For this review, take the finished solid that the model builds, in its own axes (mm). Coordinates: 2 decimals unless noted, no trailing zeros. Use a Markdown table: item, result.
from build123d import *

# Parameters (mm, degrees)
SKETCH_1_R          = 13.5
EXTRUDE_1_DEPTH     = 2
SKETCH_2_R          = 6.25
SKETCH_2_R_2        = 1.5
SKETCH_2_R_3        = 4.25
CUT_EXTRUDE_2_DEPTH = 135.372484569
SKETCH_3_R          = 1.5
CUT_EXTRUDE_3_DEPTH = 135.372484569


with BuildPart() as part:
    # 草图1 → 凸台-拉伸1 (new body)
    with BuildSketch(Plane.XY):
        Circle(SKETCH_1_R)
        with BuildLine():
            ThreePointArc((5.892711217, -11.0238811), (8.326059469, 9.323450741), (-11.617581648, 4.613219771))
            add(Edge.make_bspline(
                [(-44.514894976, -15.648119029), (-23.754992487, -12.049932399), (-11.617581648, 4.613219771)],
                knots=[0, 0, 0, 1, 1, 1], degree=2))
            add(Edge.make_bspline(
                [(-44.514894976, -15.648119029), (-60.493246192, -16.620966096), (-98.719374485, 13.99401616), (-101.099323327, 34.577284328)],
                knots=[0, 0, 0, 0, 1, 1, 1, 1], degree=3))
            ThreePointArc((-101.099323327, 34.577284328), (-119.514224633, 44.92723863), (-120.988196928, 23.854565571))
            add(Edge.make_bspline(
                [(-43.715031798, -30.941916126), (-74.6558876, -29.772176263), (-107.934743734, 0.909272839), (-120.988196928, 23.854565571)],
                knots=[0, 0, 0, 0, 1, 1, 1, 1], degree=3))
            add(Edge.make_bspline(
                [(5.892711217, -11.0238811), (-16.208282922, -27.819747246), (-43.715031798, -30.941916126)],
                knots=[0, 0, 0, 1, 1, 1], degree=2))
        make_face()
    extrude(amount=EXTRUDE_1_DEPTH)

    # 草图2 → 切除-拉伸2 (cut, through all)
    with BuildSketch(Plane.XY):
        Circle(SKETCH_2_R)
        with Locations((-7.071067812, 7.071067812)):
            Circle(SKETCH_2_R_2)
        with Locations((7.071067812, 7.071067812)):
            Circle(SKETCH_2_R_2)
        with Locations((7.071067812, -7.071067812)):
            Circle(SKETCH_2_R_2)
        with Locations((-7.071067812, -7.071067812)):
            Circle(SKETCH_2_R_2)
        with Locations((-113.582262859, 33.924428557)):
            Circle(SKETCH_2_R_3)
        with Locations((-106.728711554, 35.34880018)):
            Circle(SKETCH_2_R_2)
        with Locations((-112.157891236, 27.070877253)):
            Circle(SKETCH_2_R_2)
        with Locations((-120.435814163, 32.500056934)):
            Circle(SKETCH_2_R_2)
        with Locations((-115.006634481, 40.777979862)):
            Circle(SKETCH_2_R_2)
    extrude(amount=CUT_EXTRUDE_2_DEPTH, mode=Mode.SUBTRACT)

    # 草图3 → 切除-拉伸3 (cut, through all)
    with BuildSketch(Plane.XY):
        with Locations((-97.840235061, 9.542968429)):
            Circle(SKETCH_3_R)
        with Locations((-25.561724323, -18.05130401)):
            Circle(SKETCH_3_R)
    extrude(amount=CUT_EXTRUDE_3_DEPTH, mode=Mode.SUBTRACT)


solid = part.part
(1) For line 1 along X through (y, z) = (-1, 0.6); line 2 along X through (y, z) = (36.5, 0.9); line 3 along X through (y, z) = (7, 0.7), list the stretches that pass through material, from the lowest coordinate up.
Found:
| item | result |
|---|---|
| line 1 | x = -101.31 to -75.02, -16.3 to -6.17, 6.17 to 13.46 |
| line 2 | x = -125.81 to -116.96, -110.2 to -107.69, -105.77 to -101.35 |
| line 3 | x = -108.83 to -84.03, -11.54 to -8.57, -5.57 to 5.57, 8.57 to 11.54 |
(2) Take a section at A-A on y = 0. State how many separate pieces and enclosed holes the cut face has, plus the area to 3 significant figures.
Found:
| item | result |
|---|---|
| separate pieces | 3 |
| enclosed holes | 0 |
| area | 84.9 mm^2 |
(3) Mouldability with a two-part tool opening along Y and no side actions: class faces 1 (the face through (-67, -9, 0)), 2 (the face through (-119.2, 45.09, 0.99)), 3 (the face through (7.88, -5.81, 0.99)) as pulls with the +Y half, pulls with the -Y half, needs draft (parallel to the pull), parting line crosses it, or undercut.
Found:
| item | result |
|---|---|
| face 1 | needs draft |
| face 2 | parting line crosses it |
| face 3 | undercut |
(4) For pin 1 Ø3.5 at (x, y) = (-7.07, 7.07) entering from +Z; pin 2 Ø2.5 at (x, y) = (-115.01, 40.78) entering from -Z, all flat-tipped, find the tip position at first contact; note any pin that passes through.
Found:
| item | result |
|---|---|
| pin 1 | stops at z = 2 |
| pin 2 | passes through |
